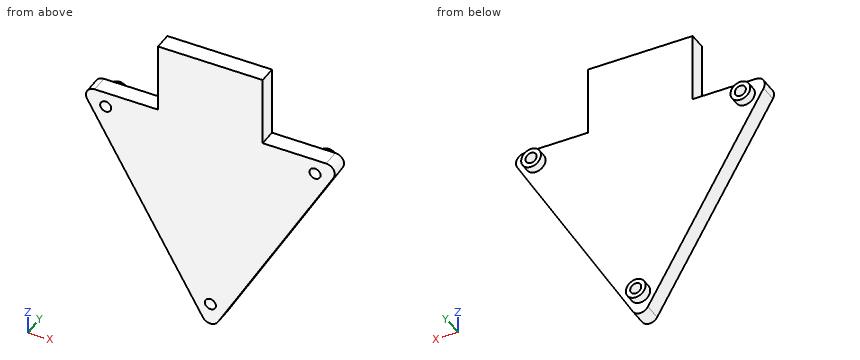
from build123d import *

# Parameters (mm, degrees)
SKETCH1_R           = 3.175
BOSS_EXTRUDE5_DEPTH = 10
SKETCH7_R           = 5.675
SKETCH7_R_2         = 3.175
BOSS_EXTRUDE7_DEPTH = 5


with BuildPart() as part:
    # Sketch1 → Boss-Extrude5 (new body)
    with BuildSketch(Plane(origin=(0, 0, 0), x_dir=(1, 0, 0), z_dir=(0, 1, 0))):
        with BuildLine():
            Line((4.330127019, 7.5), (70.669872981, 122.403810568))
            ThreePointArc((70.669872981, 122.403810568), (75, 124.903810568), (79.330127019, 122.403810568))
            Line((79.330127019, 122.403810568), (145.669872981, 7.5))
            ThreePointArc((145.669872981, 7.5), (145.669873, 2.500000033), (141.339746038, 0))
            Line((141.339746038, 0), (105.000000038, 0))
            Line((105.000000038, 0), (105.000000038, -40))
            Line((105.000000038, -40), (45.000000038, -40))
            Line((45.000000038, -40), (45.000000038, 0))
            Line((45.000000038, 0), (8.660254038, 0))
            ThreePointArc((8.660254038, 0), (4.330127019, 2.5), (4.330127019, 7.5))
        make_face()
        with Locations(Location((75, 112.583302492, 0), (0, 0, 270))):
            Circle(SKETCH1_R, mode=Mode.SUBTRACT)
        with Locations(Location((15, 8.660254038, 0), (0, 0, 270))):
            Circle(SKETCH1_R, mode=Mode.SUBTRACT)
        with Locations(Location((135, 8.660254038, 0), (0, 0, 270))):
            Circle(SKETCH1_R, mode=Mode.SUBTRACT)
    extrude(amount=BOSS_EXTRUDE5_DEPTH)

    # Sketch7 → Boss-Extrude7 (add)
    # profile 1 of 3: a face of its own
    with BuildSketch(Plane(origin=(0, 10, 0), x_dir=(1, 0, 0), z_dir=(0, 1, 0))):
        with Locations(Location((15, 8.660254038, 0), (0, 0, 270))):
            Circle(SKETCH7_R)
        with Locations(Location((15, 8.660254038, 0), (0, 0, 270))):
            Circle(SKETCH7_R_2, mode=Mode.SUBTRACT)
    # profile 2 of 3: a face of its own
    with BuildSketch(Plane(origin=(0, 10, 0), x_dir=(1, 0, 0), z_dir=(0, 1, 0))):
        with Locations(Location((135, 8.660254038, 0), (0, 0, 270))):
            Circle(SKETCH7_R)
        with Locations(Location((135, 8.660254038, 0), (0, 0, 270))):
            Circle(SKETCH7_R_2, mode=Mode.SUBTRACT)
    # profile 3 of 3: a face of its own
    with BuildSketch(Plane(origin=(0, 10, 0), x_dir=(1, 0, 0), z_dir=(0, 1, 0))):
        with Locations(Location((75, 112.583302492, 0), (0, 0, 270))):
            Circle(SKETCH7_R)
        with Locations(Location((75, 112.583302492, 0), (0, 0, 270))):
            Circle(SKETCH7_R_2, mode=Mode.SUBTRACT)
    extrude(amount=BOSS_EXTRUDE7_DEPTH)


solid = part.part
Verification items for the finished model (mm, model axes). Give positions to 0.01 mm unless a question says otherwise; leave off trailing zeros. Write each loop counter-clockwise with the first axis right and the second up, starting at its lowest first coordinate (ties: lowest second). Pieces come first, ordered by that corner, then holes. Notation, with made-up numbers: (74.5, -3) -> (99.5, -3) arc R18 cw to (99.5, 17) -> close; hole circle Ø4 at (-10, 42). An arc over 180 degrees is marked (long way). Use CSV: the item, a comma, the result in double quotes.
(1) Sectioned sample at B-B (y = 12.5). Record the cut outline in (x, z) (3 decimals), plus the area to 3 significant figures.
Derived:
outline,"circle Ø11.35 at (15, -8.66); circle Ø11.35 at (75, -112.583); circle Ø11.35 at (135, -8.66); hole circle Ø6.35 at (15, -8.66); hole circle Ø6.35 at (75, -112.583); hole circle Ø6.35 at (135, -8.66)"
area,"209 mm^2"
(2) Go/stop test with flat-tipped pins: pin 1 (7.5 mm diameter, centred on x = 135, z = -8.66, fed in from +Y); pin 2 (8 mm diameter, centred on x = 129.5, y = 6, fed in from +Z); pin 3 (5 mm diameter, centred on x = 15, z = -8.66, fed in from +Y); pin 4 (3 mm diameter, centred on y = 6.5, z = 20.5, fed in from -X). Record where each tip stops, or that it passes through.
Derived:
pin 1,"stops at y = 15"
pin 2,"stops at z = 0"
pin 3,"passes through"
pin 4,"stops at x = 45"
(3) Sectioned sample at C-C (y = 2). Record the cut outline in (x, z) (3 decimals), plus the area to 3 significant figures.
Derived:
outline,"(4.33, -7.5) -> (70.67, -122.404) arc R5 ccw to (79.33, -122.404) -> (145.67, -7.5) arc R5 ccw to (141.34, 0) -> (105, 0) -> (105, 40) -> (45, 40) -> (45, 0) -> (8.66, 0) arc R5 ccw to start; hole circle Ø6.35 at (15, -8.66); hole circle Ø6.35 at (75, -112.583); hole circle Ø6.35 at (135, -8.66)"
area,"12,000 mm^2"
(4) Sectioned sample at D-D (z = 28.5). Record the cut outline in (x, y), plus the area to 3 significant figures.
Derived:
outline,"(45, 0) -> (105, 0) -> (105, 10) -> (45, 10) -> close"
area,"600 mm^2"
(5) Sectioned sample at A-A (x = 75). Record the cut outline in (y, z), plus the area to 3 significant figures.
Derived:
outline,"(0, -124.9) -> (10, -124.9) -> (10, -118.26) -> (15, -118.26) -> (15, -115.76) -> (0, -115.76) -> close; (0, -109.41) -> (15, -109.41) -> (15, -106.91) -> (10, -106.91) -> (10, 40) -> (0, 40) -> close"
area,"1,610 mm^2"
(6) Material ranges on L1, parallel to Y at x = 56, z = -36; L2, parallel to X at y = 2.75, z = -113; L3, parallel to X at y = 4.5, z = 15, recorded low to high.
Derived:
L1,"y = 0 to 10"
L2,"x = 65.24 to 71.85, 78.15 to 84.76"
L3,"x = 45 to 105"
